```python
from build123d import *

# Parameters (mm, degrees)
SKETCH2_W               = 170
SKETCH2_H               = 170
BOSS_EXTRUDE1_DEPTH     = 10
CUT_EXTRUDE2_DEPTH      = 121.623380818
CUT_EXTRUDE2_DEPTH_BACK = 121.623380818
SKETCH4_R               = 1.5
SKETCH6_R               = 2.5
CUT_EXTRUDE6_DEPTH      = 10


with BuildPart() as part:
    # Sketch2 → Boss-Extrude1 (new body)
    with BuildSketch(Plane(origin=(0, 0, 0), x_dir=(1, 0, 0), z_dir=(0, 1, 0))):
        Rectangle(SKETCH2_W, SKETCH2_H)
    extrude(amount=BOSS_EXTRUDE1_DEPTH)

    # Sketch4 → Cut-Extrude2 (cut, two sides: drawn at the far end of the back side and taken through both)
    with BuildSketch(Plane(origin=(0, 0, 0), x_dir=(-1, 0, 0), z_dir=(0, -1, 0)).offset(-CUT_EXTRUDE2_DEPTH_BACK)):
        with Locations(Location((-70.33, -9, 0), (0, 0, 270))):
            Circle(SKETCH4_R)
        with Locations(Location((-70.33, 9, 0), (0, 0, 270))):
            Circle(SKETCH4_R)
        with Locations(Location((70.33, 9, 0), (0, 0, 270))):
            Circle(SKETCH4_R)
        with Locations(Location((70.33, -9, 0), (0, 0, 270))):
            Circle(SKETCH4_R)
        with Locations(Location((46.4, 9, 0), (0, 0, 270))):
            Circle(SKETCH4_R)
        with Locations(Location((46.4, -9, 0), (0, 0, 270))):
            Circle(SKETCH4_R)
        with Locations(Location((-46.4, -9, 0), (0, 0, 270))):
            Circle(SKETCH4_R)
        with Locations(Location((-46.4, 9, 0), (0, 0, 270))):
            Circle(SKETCH4_R)
    extrude(amount=CUT_EXTRUDE2_DEPTH + CUT_EXTRUDE2_DEPTH_BACK, mode=Mode.SUBTRACT)

    # Sketch6 → Cut-Extrude6 (cut)
    with BuildSketch(Plane.XZ):
        with Locations(Location((-15.68, 0, 0), (0, 0, 270))):
            Circle(SKETCH6_R)
        with Locations(Location((15.68, 0, 0), (0, 0, 270))):
            Circle(SKETCH6_R)
    extrude(amount=-CUT_EXTRUDE6_DEPTH, mode=Mode.SUBTRACT)


solid = part.part
```
Geometry check sheet. Reference: the model listing, model coordinates, mm. Coordinates: 2 decimals unless noted, no trailing zeros. Loops run counter-clockwise (first coordinate to the right, second up) from the corner with the lowest first, then second, coordinate; pieces in that order, holes last. Notation, with made-up numbers: (14.5, 50.5) - (69.5, 50.5) arc R12 ccw to (69.5, 61.5) - close; hole circle Ø5 at (77, 89). An arc over 180 degrees is marked (long way). One line per item, written item: value. Start each with the question number.
(1) Cross-section at A-A on x = -15.68. Enter the section's corners in (y, z), plus the area to 3 significant figures.
(2) Material ranges on line 1 (X direction, y = 7, z = 9); line 2 (Z direction, x = -70.33, y = 4.25); line 3 (Z direction, x = 17.5, y = 8.5), recorded low to high. Write a range as [from, to].
(3) Mould release check, pull along X, two halves, no side actions. Record for faces 1 (the flat face through (-85, 5, 1)), 2 (the flat face through (85, 5, 1)), 3 (the cylindrical face through (-13.2, 4.9, 0.3)), 4 (the flat face through (-1, 10, -1)): released by +X, released by -X, zero draft, split by the parting line, or undercut.
Results below:
1. outline: (0, -85) - (10, -85) - (10, -2.5) - (0, -2.5) - close; (0, 2.5) - (10, 2.5) - (10, 85) - (0, 85) - close
1. area: 1,650 mm2
2. line 1: x = [-85, -71.83], [-68.83, -47.9], [-44.9, 44.9], [47.9, 68.83], [71.83, 85]
2. line 2: z = [-85, -10.5], [-7.5, 7.5], [10.5, 85]
2. line 3: z = [-85, -1.71], [1.71, 85]
3. face 1: released by -X
3. face 2: released by +X
3. face 3: undercut
3. face 4: zero draft
